CAD build for the part. Positions are in the model's coordinates, mm. Face numbers are marked on the shaded views. A direction names the side the tool comes from. Give positions to 0.01 mm unless a question says otherwise; leave off trailing zeros. Loops run counter-clockwise (first coordinate to the right, second up) from the corner with the lowest first, then second, coordinate; pieces in that order, holes last.
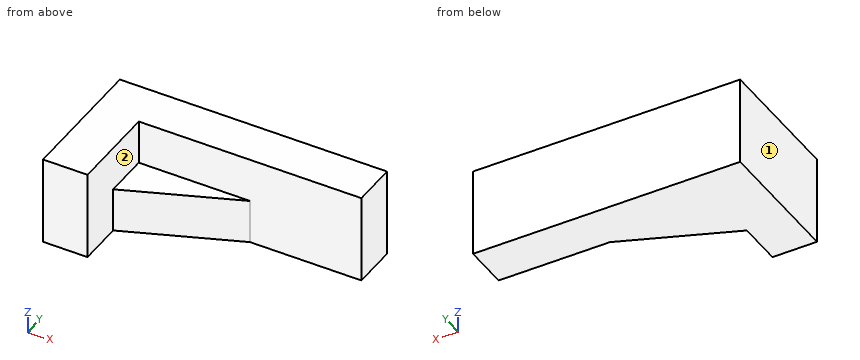
```python
from build123d import *

# Parameters (mm, degrees)
F0_W     = 152.4
F0_H     = 50.8
F1_DEPTH = 76.2
F3_DEPTH = 50.8
F4_DEPTH = 25.4


with BuildPart() as f1:
    # F0 (on Front) → F1 (new body)
    with BuildSketch(Plane.XZ):
        with Locations((76.2, 25.4)):
            Rectangle(F0_W, F0_H)
    extrude(amount=F1_DEPTH)

    # F2 (on face) → F3 (cut)
    with BuildSketch(Plane.XY.offset(50.8)):
        Polygon((25.4, -50.8), (25.4, -76.2), (152.4, -76.2), (152.4, -25.4), (88.9, -25.4), align=None)
    extrude(amount=-F3_DEPTH, mode=Mode.SUBTRACT)

    # F2 (on face) → F4 (cut)
    with BuildSketch(Plane.XY.offset(50.8)):
        Polygon((25.4, -25.4), (25.4, -50.8), (88.9, -25.4), align=None)
    extrude(amount=-F4_DEPTH, mode=Mode.SUBTRACT)


solid = f1.part
```
1. Probe line 1 along X through (y, z) = (-66.5, 11.5); line 2 along Y through (x, z) = (38, 27). List the from-to ranges inside material, lowest first.
Responses:
line 1: x = 0 to 25.4
line 2: y = -25.4 to 0
2. Saw through at A-A, the plane z = 6. List the corners of the cut face in (x, y), and give its area (3 significant figures).
Responses:
outline: (0, -76.2) - (25.4, -76.2) - (25.4, -50.8) - (88.9, -25.4) - (152.4, -25.4) - (152.4, 0) - (0, 0) - close
area: 5,970 mm2
3. Saw through at B-B, the plane y = -37. List the corners of the cut face in (x, z), and give its area (3 significant figures).
Responses:
outline: (0, 0) - (59.9, 0) - (59.9, 25.4) - (25.4, 25.4) - (25.4, 50.8) - (0, 50.8) - close
area: 2,170 mm2
4. Drop flat-ended pins along their axis: pin 1 (20.5 mm diameter, centred on x = 42.5, y = -40.5, fed in from +Z); pin 2 (10 mm diameter, centred on x = 31, z = 21.5, fed in from -Y); pin 3 (15 mm diameter, centred on x = 64.5, z = 13.5, fed in from -Y). Give the stop position or say it passes through.
Responses:
pin 1: stops at z = 25.4
pin 2: stops at y = -50.56
pin 3: stops at y = -38.16
5. Tool access for the marked faces 1 and 2: list every direction of +Z, -Z, +X, -X, +Y, -Y with a clear straight run to the whole face (end or side of a thin tool).
Responses:
face 1: +Z, -Z, -X, +Y, -Y
face 2: +Z, +X, -Y
6. Saw through at D-D, the plane x = 98. List the corners of the cut face in (y, z).
Responses:
outline: (-25.4, 0) - (0, 0) - (0, 50.8) - (-25.4, 50.8) - close
7. Saw through at C-C, the plane x = 46.5. List the corners of the cut face in (y, z), and give its area (3 significant figures).
Responses:
outline: (-42.36, 0) - (0, 0) - (0, 50.8) - (-25.4, 50.8) - (-25.4, 25.4) - (-42.36, 25.4) - close
area: 1,720 mm2
